Geometry check sheet. Reference: the model listing, model coordinates, mm. A direction names the side the tool comes from. Round coordinates to 2 decimals unless told otherwise and drop trailing zeros. Loops run counter-clockwise (first coordinate to the right, second up) from the corner with the lowest first, then second, coordinate; pieces in that order, holes last. Notation, with made-up numbers: M 82,25.5 L 139,25.5 A19 cw 139,38.5 Z; hole C 27.5,24.5 d1. An arc over 180 degrees is marked long. Use one line per item in the form item = value. Start each with the question number.
1. Go/stop test with flat-tipped pins: pin 1 (2 mm diameter, centred on y = -2.5, z = 39.5, fed in from +X); pin 2 (1.2 mm diameter, centred on x = -21.5, y = -2, fed in from -Z); pin 3 (4.5 mm diameter, centred on x = 9, z = 45, fed in from -Y); pin 4 (3 mm diameter, centred on x = -9, z = 45, fed in from +Y). Record where each tip stops, or that it passes through.
2. Cross-section at C-C (z = 21). Record the boundary of the cut face in (x, y).
3. Material ranges on line 1 (Z direction, x = -9, y = -2.5); line 2 (X direction, y = -1.7, z = 45); line 3 (Z direction, x = 9.5, y = -3.6), recorded low to high.
4. Set-up check for faces 3 (the flat face through (0.155, 0.986, 31.229)), 4 (the flat face through (-1, -2, 13.35)), 5 (the cylindrical face through (5.831, 0.986, 25.043)): record each of +Z, -Z, +X, -X, +Y, -Y from which the full face is reachable in a straight line by a thin tool's end or side.
5. Cross-section at B-B (y = -1.65). State how many separate pieces and enclosed holes the cut face has, then the cut area to 3 significant figures.
6. Cross-section at A-A (x = -9). Record the boundary of the cut face in (y, z), then the cut area to 3 significant figures.
7. Cross-section at D-D (x = -26). Record the boundary of the cut face in (y, z), then the cut area to 3 significant figures.
8. Draft check along Z on faces 1 (the flat face through (-10, 1, 37.027)), 2 (the flat face through (6, 1, 37.027)). Enter one of: pulls with the +Z half, pulls with the -Z half, needs draft (parallel to the pull), parting line crosses it, or undercut.
```python
from build123d import *

# Parameters (mm, degrees)
F4_DEPTH = 4
F0_R     = 1.75
F5_DEPTH = 25
F7_DEPTH = 2


with BuildPart() as f4:
    # F3 (on Front) → F4 (new body)
    with BuildSketch(Plane.XZ):
        Polygon((14.7063490003, 20.4016491771), (14.4608622171, 48.8), (-13.3913809769, 48.8), (-31.4313102054, 34.6867430935), (-31.4313102054, 17.5032976646), (-12.7962362449, 8), (21.2817378342, 8), (21.2817378342, 15.3483422473), align=None)
    extrude(amount=F4_DEPTH)

    # F0 (on Front) + F1 (on Front) + F2 (on Front) → F5 (cut)
    with BuildSketch(Plane.XZ):
        with Locations((-9, 45)):
            Circle(F0_R)
        with Locations((9, 45)):
            Circle(F0_R)
    with BuildSketch(Plane.XZ):
        with BuildLine():
            Line((10.5241951349, 10.7379024326), (12, 10))
            Line((12, 10), (13.65, 10))
            ThreePointArc((13.65, 10), (13.4035738338, 10.867456335), (12.7379024326, 11.4758048651))
            Line((12.7379024326, 11.4758048651), (12.3895121629, 11.65))
            Line((12.3895121629, 11.65), (12, 11.65))
            ThreePointArc((12, 11.65), (11.132543665, 11.4035738338), (10.5241951349, 10.7379024326))
        make_face()
        with BuildLine():
            Line((13.65, 10), (12, 10))
            Line((12, 10), (10.5241951349, 10.7379024326))
            ThreePointArc((10.5241951349, 10.7379024326), (10.4346725582, 9.4782241861), (11.2620975674, 8.5241951349))
            ThreePointArc((11.2620975674, 8.5241951349), (11.6209076811, 8.3941391674), (12, 8.35))
            ThreePointArc((12, 8.35), (13.166726189, 8.833273811), (13.65, 10))
        make_face()
        with BuildLine():
            ThreePointArc((12.7379024326, 11.4758048651), (13.4035738338, 10.867456335), (13.65, 10))
            ThreePointArc((13.65, 10), (13.166726189, 8.833273811), (12, 8.35))
            Line((12, 8.35), (17, 8.35))
            ThreePointArc((17, 8.35), (18.65, 10), (17, 11.65))
            Line((17, 11.65), (12.3895121629, 11.65))
            Line((12.3895121629, 11.65), (12.7379024326, 11.4758048651))
        make_face()
        with BuildLine():
            ThreePointArc((11.2620975674, 8.5241951349), (10.4346725582, 9.4782241861), (10.5241951349, 10.7379024326))
            Line((10.5241951349, 10.7379024326), (3.4758048651, 14.2620975674))
            ThreePointArc((3.4758048651, 14.2620975674), (2.867456335, 13.5964261662), (2, 13.35))
            Line((2, 13.35), (1.6104878371, 13.35))
            Line((1.6104878371, 13.35), (11.2620975674, 8.5241951349))
        make_face()
        with BuildLine():
            Line((3.4758048651, 14.2620975674), (10.5241951349, 10.7379024326))
            ThreePointArc((10.5241951349, 10.7379024326), (11.132543665, 11.4035738338), (12, 11.65))
            Line((12, 11.65), (12.3895121629, 11.65))
            Line((12.3895121629, 11.65), (2.7379024326, 16.4758048651))
            ThreePointArc((2.7379024326, 16.4758048651), (3.5653274418, 15.5217758139), (3.4758048651, 14.2620975674))
        make_face()
        with BuildLine():
            ThreePointArc((2, 13.35), (2.867456335, 13.5964261662), (3.4758048651, 14.2620975674))
            Line((3.4758048651, 14.2620975674), (2, 15))
            Line((2, 15), (0.35, 15))
            ThreePointArc((0.35, 15), (0.5964261662, 14.132543665), (1.2620975674, 13.5241951349))
            Line((1.2620975674, 13.5241951349), (1.6104878371, 13.35))
            Line((1.6104878371, 13.35), (2, 13.35))
        make_face()
        with BuildLine():
            Line((2, 15), (3.4758048651, 14.2620975674))
            ThreePointArc((3.4758048651, 14.2620975674), (3.5653274418, 15.5217758139), (2.7379024326, 16.4758048651))
            ThreePointArc((2.7379024326, 16.4758048651), (2.3790923189, 16.6058608326), (2, 16.65))
            ThreePointArc((2, 16.65), (0.833273811, 16.166726189), (0.35, 15))
            Line((0.35, 15), (2, 15))
        make_face()
        with BuildLine():
            Line((-3, 13.35), (1.6104878371, 13.35))
            Line((1.6104878371, 13.35), (1.2620975674, 13.5241951349))
            ThreePointArc((1.2620975674, 13.5241951349), (0.5964261662, 14.132543665), (0.35, 15))
            ThreePointArc((0.35, 15), (0.833273811, 16.166726189), (2, 16.65))
            Line((2, 16.65), (-3, 16.65))
            ThreePointArc((-3, 16.65), (-4.65, 15), (-3, 13.35))
        make_face()
    with BuildSketch(Plane.XZ):
        with BuildLine():
            Line((-11.4758048651, 21.7379024326), (-10, 21))
            Line((-10, 21), (-8.35, 21))
            ThreePointArc((-8.35, 21), (-8.5964261662, 21.867456335), (-9.2620975674, 22.4758048651))
            Line((-9.2620975674, 22.4758048651), (-9.6104878371, 22.65))
            Line((-9.6104878371, 22.65), (-10, 22.65))
            ThreePointArc((-10, 22.65), (-10.867456335, 22.4035738338), (-11.4758048651, 21.7379024326))
        make_face()
        with BuildLine():
            Line((-8.35, 21), (-10, 21))
            Line((-10, 21), (-11.4758048651, 21.7379024326))
            ThreePointArc((-11.4758048651, 21.7379024326), (-11.5653274418, 20.4782241861), (-10.7379024326, 19.5241951349))
            ThreePointArc((-10.7379024326, 19.5241951349), (-10.3790923189, 19.3941391674), (-10, 19.35))
            ThreePointArc((-10, 19.35), (-8.833273811, 19.833273811), (-8.35, 21))
        make_face()
        with BuildLine():
            ThreePointArc((-9.2620975674, 22.4758048651), (-8.5964261662, 21.867456335), (-8.35, 21))
            ThreePointArc((-8.35, 21), (-8.833273811, 19.833273811), (-10, 19.35))
            Line((-10, 19.35), (-5, 19.35))
            ThreePointArc((-5, 19.35), (-3.35, 21), (-5, 22.65))
            Line((-5, 22.65), (-9.6104878371, 22.65))
            Line((-9.6104878371, 22.65), (-9.2620975674, 22.4758048651))
        make_face()
        with BuildLine():
            ThreePointArc((-10.7379024326, 19.5241951349), (-11.5653274418, 20.4782241861), (-11.4758048651, 21.7379024326))
            Line((-11.4758048651, 21.7379024326), (-18.5241951349, 25.2620975674))
            ThreePointArc((-18.5241951349, 25.2620975674), (-19.132543665, 24.5964261662), (-20, 24.35))
            Line((-20, 24.35), (-20.3895121629, 24.35))
            Line((-20.3895121629, 24.35), (-10.7379024326, 19.5241951349))
        make_face()
        with BuildLine():
            Line((-18.5241951349, 25.2620975674), (-11.4758048651, 21.7379024326))
            ThreePointArc((-11.4758048651, 21.7379024326), (-10.867456335, 22.4035738338), (-10, 22.65))
            Line((-10, 22.65), (-9.6104878371, 22.65))
            Line((-9.6104878371, 22.65), (-19.2620975674, 27.4758048651))
            ThreePointArc((-19.2620975674, 27.4758048651), (-18.4346725582, 26.5217758139), (-18.5241951349, 25.2620975674))
        make_face()
        with BuildLine():
            ThreePointArc((-20, 24.35), (-19.132543665, 24.5964261662), (-18.5241951349, 25.2620975674))
            Line((-18.5241951349, 25.2620975674), (-20, 26))
            Line((-20, 26), (-21.65, 26))
            ThreePointArc((-21.65, 26), (-21.4035738338, 25.132543665), (-20.7379024326, 24.5241951349))
            Line((-20.7379024326, 24.5241951349), (-20.3895121629, 24.35))
            Line((-20.3895121629, 24.35), (-20, 24.35))
        make_face()
        with BuildLine():
            Line((-20, 26), (-18.5241951349, 25.2620975674))
            ThreePointArc((-18.5241951349, 25.2620975674), (-18.4346725582, 26.5217758139), (-19.2620975674, 27.4758048651))
            ThreePointArc((-19.2620975674, 27.4758048651), (-19.6209076811, 27.6058608326), (-20, 27.65))
            ThreePointArc((-20, 27.65), (-21.166726189, 27.166726189), (-21.65, 26))
            Line((-21.65, 26), (-20, 26))
        make_face()
        with BuildLine():
            Line((-25, 24.35), (-20.3895121629, 24.35))
            Line((-20.3895121629, 24.35), (-20.7379024326, 24.5241951349))
            ThreePointArc((-20.7379024326, 24.5241951349), (-21.4035738338, 25.132543665), (-21.65, 26))
            ThreePointArc((-21.65, 26), (-21.166726189, 27.166726189), (-20, 27.65))
            Line((-20, 27.65), (-25, 27.65))
            ThreePointArc((-25, 27.65), (-26.65, 26), (-25, 24.35))
        make_face()
    extrude(amount=F5_DEPTH, mode=Mode.SUBTRACT)

    # F6 (on face) → F7 (join)
    with BuildSketch(Plane(origin=(0, 0, 0), x_dir=(-1, 0, 0), z_dir=(0, 1, 0))):
        with BuildLine():
            Line((0.9742605893, 39.5259801518), (0.4651322738, 38.6772193015))
            Line((0.4651322738, 38.6772193015), (2.3892181925, 38.6772193015))
            Line((2.3892181925, 38.6772193015), (4.0392181925, 38.6772193015))
            ThreePointArc((4.0392181925, 38.6772193015), (3.5559443815, 39.8439454904), (2.3892181925, 40.3272193015))
            ThreePointArc((2.3892181925, 40.3272193015), (1.5761854143, 40.1130040003), (0.9742605893, 39.5259801518))
        make_face()
        with BuildLine():
            Line((-0.5246185145, 37.0272193015), (0.4651322738, 38.6772193015))
            Line((0.4651322738, 38.6772193015), (0.9742605893, 39.5259801518))
            ThreePointArc((0.9742605893, 39.5259801518), (1.5761854143, 40.1130040003), (2.3892181925, 40.3272193015))
            Line((2.3892181925, 40.3272193015), (-11.0781090334, 40.3272193015))
            ThreePointArc((-11.0781090334, 40.3272193015), (-12.7281090334, 38.6772193015), (-11.0781090334, 37.0272193015))
            Line((-11.0781090334, 37.0272193015), (-0.5246185145, 37.0272193015))
        make_face()
        Polygon((2.3892181925, 38.6772193015), (0.4651322738, 38.6772193015), (-0.5246185145, 37.0272193015), (1.3994674043, 37.0272193015), align=None)
        with BuildLine():
            Line((4.0392181925, 38.6772193015), (2.3892181925, 38.6772193015))
            Line((2.3892181925, 38.6772193015), (1.3994674043, 37.0272193015))
            Line((1.3994674043, 37.0272193015), (3.3235533231, 37.0272193015))
            Line((3.3235533231, 37.0272193015), (3.8041757958, 37.8284584511))
            ThreePointArc((3.8041757958, 37.8284584511), (3.9793722803, 38.2368671954), (4.0392181925, 38.6772193015))
        make_face()
        with BuildLine():
            Line((1.3994674043, 37.0272193015), (-0.5246185145, 37.0272193015))
            Line((-0.5246185145, 37.0272193015), (-6.3666907677, 27.2879805636))
            ThreePointArc((-6.3666907677, 27.2879805636), (-5.8004940149, 25.02426211), (-3.5367755613, 25.5904588628))
            Line((-3.5367755613, 25.5904588628), (3.3235533231, 37.0272193015))
            Line((3.3235533231, 37.0272193015), (1.3994674043, 37.0272193015))
        make_face()
        with BuildLine():
            ThreePointArc((2.3892181925, 40.3272193015), (3.5559443815, 39.8439454904), (4.0392181925, 38.6772193015))
            ThreePointArc((4.0392181925, 38.6772193015), (3.9793722803, 38.2368671954), (3.8041757958, 37.8284584511))
            Line((3.8041757958, 37.8284584511), (3.3235533231, 37.0272193015))
            Line((3.3235533231, 37.0272193015), (17.1748909666, 37.0272193015))
            ThreePointArc((17.1748909666, 37.0272193015), (18.8248909666, 38.6772193015), (17.1748909666, 40.3272193015))
            Line((17.1748909666, 40.3272193015), (2.3892181925, 40.3272193015))
        make_face()
    extrude(amount=F7_DEPTH)


solid = f4.part
```
Reported:
q1.pin_1 = 14.55
q1.pin_2 = 12.13
q1.pin_3 = -4
q1.pin_4 = through
q2.outline = M -31.43,-4 L -13.69,-4 L -13.69,0 L -31.43,0 Z; M -3.35,-4 L 14.7,-4 L 14.7,0 L -3.35,0 Z
q3.line_1 = 8 to 19.35, 22.65 to 43.25, 46.75 to 48.8
q3.line_2 = -18.25 to -10.75, -7.25 to 7.25, 10.75 to 14.49
q3.line_3 = 8 to 9.41, 13.09 to 43.32, 46.68 to 48.8
q4.face_3 = -Z, -X, +Y
q4.face_4 = +Y, -Y
q4.face_5 = +Y
q5.separate_pieces = 1
q5.enclosed_holes = 4
q5.area = 1,550 mm²
q6.outline = M -4,8 L 0,8 L 0,19.35 L -4,19.35 Z; M -4,22.65 L 0,22.65 L 0,37.03 L 2,37.03 L 2,40.33 L 0,40.33 L 0,43.25 L -4,43.25 Z; M -4,46.75 L 0,46.75 L 0,48.8 L -4,48.8 Z
q6.area = 143 mm²
q7.outline = M -4,14.73 L 0,14.73 L 0,24.69 L -4,24.69 Z; M -4,27.31 L 0,27.31 L 0,38.94 L -4,38.94 Z
q7.area = 86.3 mm²
q8.face_1 = pulls with the -Z half
q8.face_2 = undercut
